Autodesk Inventor part; units mm, degrees
ref_plane "YZ Plane" through (0, 0, 0) normal (1, 0, 0) x (0, 1, 0)
ref_plane "XZ Plane" through (0, 0, 0) normal (0, 1, 0) x (-1, 0, 0)
ref_plane "XY Plane" through (0, 0, 0) normal (0, 0, 1) x (1, 0, 0)
sketch "Sketch1" plane through (0, 0, 0) normal (0, 1, 0) x (-1, 0, 0)
  line L0 (6.5, -3.7528) -> (0, -7.5056)
  line L1 (0, -7.5056) -> (-6.5, -3.7528)
  line L2 (-6.5, -3.7528) -> (-6.5, 3.7528)
  line L3 (-6.5, 3.7528) -> (0, 7.5056)
  line L4 (0, 7.5056) -> (6.5, 3.7528)
  line L5 (6.5, 3.7528) -> (6.5, -3.7528)
  circle A0 centre (0, 0) radius 4
  point P0 (6.5, 0)
  dimension "d0" = 13
  dimension "d3" = 8
extrude "Extrusion1" add sketch "Sketch1" along normal blind 5
chamfer "Chamfer1" distance 0.8 angle 45 12 edges at (-3.25, 5, 5.6292) (-6.5, 5, 0) (-3.25, 5, -5.6292) (3.25, 5, -5.6292) (6.5, 5, 0) (3.25, 5, 5.6292) (-3.25, 0, 5.6292) (3.25, 0, 5.6292) (6.5, 0, 0) (3.25, 0, -5.6292) (-3.25, 0, -5.6292) (-6.5, 0, 0)
properties part number "M8_Nut"
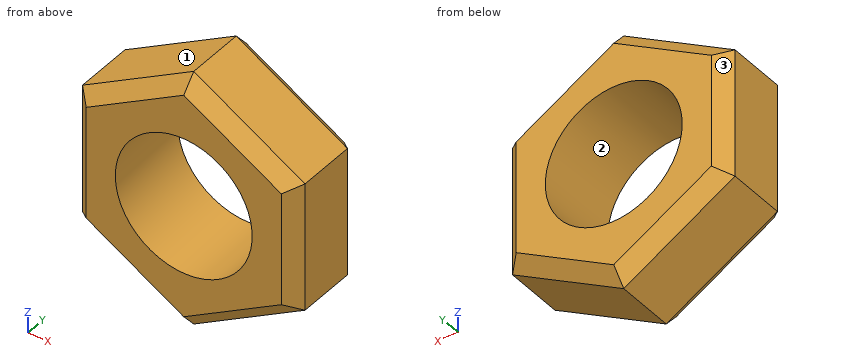
Part model, mm, in its own coordinate system. Face numbers are marked on the shaded views. Round coordinates to 2 decimals unless told otherwise and drop trailing zeros. Loops run counter-clockwise (first coordinate to the right, second up) from the corner with the lowest first, then second, coordinate; pieces in that order, holes last. Notation, with made-up numbers: (35.25, 68) -> (59.25, 68) arc R21 ccw to (59.25, 94) -> close; hole circle Ø4 at (84.25, 8). An arc over 180 degrees is marked (long way). Use one line per item in the form item = value. Start each with the question number.
Item 1: Band-saw the part on B-B (y = 1.8). List the corners of the cut face in (x, z), plus the area to 3 significant figures.
Item 2: Band-saw the part on A-A (z = 0). List the corners of the cut face in (x, y).
Item 3: Band-saw the part on C-C (x = 1.75). List the corners of the cut face in (y, z), plus the area to 3 significant figures.
Item 4: Drill centre lines: line 1 along Z through (x, y) = (3.5, 1.9); line 2 along X through (y, z) = (3.05, -2.75); line 3 along X through (y, z) = (1.75, -1.5). Where is each one in solid material? Low to high.
Item 5: Two-plate mould, pull along Z, no slides. Class the marked faces 1, 2 and 3: released by +Z, released by -Z, zero draft, split by the parting line, or undercut.
Item 6: Band-saw the part on D-D (x = -4.5). List the corners of the cut face in (y, z), plus the area to 3 significant figures.
Data:
q1.outline = (-6.5, -3.75) -> (0, -7.51) -> (6.5, -3.75) -> (6.5, 3.75) -> (0, 7.51) -> (-6.5, 3.75) -> close; hole circle Ø8 at (0, 0)
q1.area = 96.1 mm^2
q2.outline = (-6.5, 0.8) -> (-5.7, 0) -> (-4, 0) -> (-4, 5) -> (-5.7, 5) -> (-6.5, 4.2) -> close; (4, 0) -> (5.7, 0) -> (6.5, 0.8) -> (6.5, 4.2) -> (5.7, 5) -> (4, 5) -> close
q3.outline = (0, -5.57) -> (0.8, -6.5) -> (4.2, -6.5) -> (5, -5.57) -> (5, -3.6) -> (0, -3.6) -> close; (0, 3.6) -> (5, 3.6) -> (5, 5.57) -> (4.2, 6.5) -> (0.8, 6.5) -> (0, 5.57) -> close
q3.area = 27.5 mm^2
q4.line_1 = -5.48 to -1.94, 1.94 to 5.48
q4.line_2 = -6.5 to -2.9, 2.9 to 6.5
q4.line_3 = -6.5 to -3.71, 3.71 to 6.5
q5.face_1 = released by +Z
q5.face_2 = undercut
q5.face_3 = zero draft
q6.outline = (0, -3.98) -> (0.8, -4.91) -> (4.2, -4.91) -> (5, -3.98) -> (5, 3.98) -> (4.2, 4.91) -> (0.8, 4.91) -> (0, 3.98) -> close
q6.area = 47.6 mm^2
